Geometry: see drawing. Coordinates: mm, zero at the bounding-box minimum. Round coordinates to 2 decimals unless told otherwise and drop trailing zeros.
(1) First-contact query: pin 1 Ø8 at (y, z) = (17, 10.5) entering from +X; pin 2 Ø6 at (y, z) = (9, 54) entering from +X; pin 3 Ø1 at (x, y) = (17.5, 16.5) entering from -Z (1 decimal). Flat tips, straight axial feed; report the tip coordinate or a pass-through.
(2) Mould query, pull axis X, two halves, no side actions, for the marked faces 1, 2 and 3. Classes: pulls with the +X half, pulls with the -X half, needs draft (parallel to the pull), parting line crosses it, or undercut.
(3) Material intervals for probe 1 along X at (y, z) = (16, 34.5) (1 decimal); probe 2 along X at (y, z) = (13.75, 43.5) (1 decimal); probe 3 along Z at (x, y) = (45.5, 11.25) (1 decimal), sorted ascending.
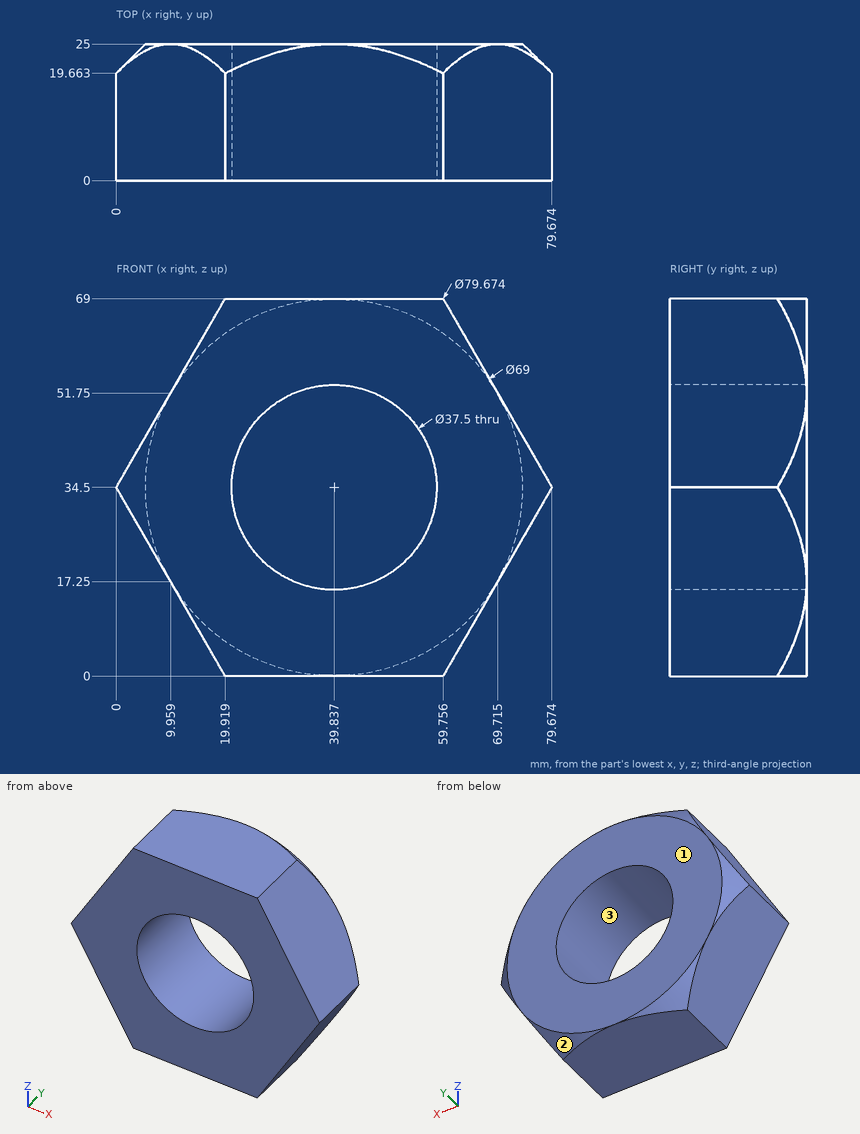
Output values:
1. pin 1: stops at x = 68.13
1. pin 2: stops at x = 70.15
1. pin 3: stops at z = 3.3
2. face 1: needs draft
2. face 2: pulls with the +X half
2. face 3: undercut
3. probe 1: x = 0 to 21.1, 58.6 to 79.7
3. probe 2: x = 5.2 to 23.4, 56.3 to 74.5
3. probe 3: z = 0 to 16.6, 52.4 to 69
